Geometry check sheet. Reference: the model listing, model coordinates, mm. A direction names the side the tool comes from. Coordinates: 2 decimals unless noted, no trailing zeros. Write each loop counter-clockwise with the first axis right and the second up, starting at its lowest first coordinate (ties: lowest second). Pieces come first, ordered by that corner, then holes. Notation, with made-up numbers: (44, 54.25) -> (74, 54.25) arc R24 ccw to (74, 90.25) -> close; hole circle Ø11 at (33, 19.5). An arc over 180 degrees is marked (long way). Answer in a Markdown table with one row per item. Add a question column.
1. Cross-section at B-B on y = 5. Record the cut outline in (x, z) (3 decimals), and give its area (3 significant figures).
2. Cross-section at D-D on y = 28.5. Record the cut outline in (x, z) (3 decimals).
3. Cross-section at A-A on x = 0. Record the cut outline in (y, z) (3 decimals), and give its area (3 significant figures).
4. Mould release check, pull along X, two halves, no side actions. Record for faces 1 (the flat face through (0, 22.225, 136)), 2 (the flat face through (-1, 26, 0)), 3 (the flat face through (38.1, 38.1, 136.3)): pulls with the +X half, pulls with the -X half, needs draft (parallel to the pull), parting line crosses it, or undercut.
5. Cross-section at C-C on z = 114. Record the cut outline in (x, y) (3 decimals), and give its area (3 significant figures).
6. Depth check by flat-ended pin: P1, Ø8, axis at x = -28.575, z = 12.7, coming from the +Y side; P2, Ø7.5, axis at x = 3, z = 13.5, coming from the -Y side (3 decimals); P3, Ø24.5, axis at x = 32.5, z = 91, coming from the +Y side. Enter the tip coordinate at first touch or a pass-through.
7. Set-up check for faces 4 (the flat face through (41.275, 9, 74)), 5 (the cylindrical face through (30.318, 14.511, 121.915)), 6 (the flat face through (0, 22.225, 13)): record each of +Z, -Z, +X, -X, +Y, -Y from which the full face is reachable in a straight line by a thin tool's end or side.
8. Scan lines: L1, parallel to Z at x = 29, y = 7 (3 decimals); L2, parallel to Z at x = 28.5, y = 31 (3 decimals); L3, parallel to X at y = 5, z = 66 (3 decimals). Record each from-to range of solid material in increasing order. Write a range as from..to.
```python
from build123d import *

# Parameters (mm, degrees)
BOSS_EXTRUDE1_DEPTH     = 149.225
CHAMFER1_SIZE           = 6.35
F_3_8_CLEARANCE_HOLE1_D = 9.8044
SKETCH4_W               = 98.425
SKETCH4_H               = 28.575
CUT_EXTRUDE1_DEPTH      = 176.460048872
FILLET1_R               = 6.35
CUT_EXTRUDE2_START      = -123.825
SKETCH5_R               = 4.500000017
CUT_EXTRUDE2_DEPTH      = 40.64


with BuildPart() as part:
    # Sketch1 → Boss-Extrude1 (new body)
    with BuildSketch(Plane.XY):
        with BuildLine():
            Line((-19.05, 0), (-19.05, 19.05))
            ThreePointArc((-19.05, 19.05), (-18.12006403, 21.29506403), (-15.875, 22.225))
            Line((-15.875, 22.225), (15.875, 22.225))
            ThreePointArc((15.875, 22.225), (18.12006403, 21.29506403), (19.05, 19.05))
            Line((19.05, 19.05), (19.05, 0))
            Line((19.05, 0), (41.275, 0))
            Line((41.275, 0), (41.275, 41.275))
            Line((41.275, 41.275), (-41.275, 41.275))
            Line((-41.275, 41.275), (-41.275, 0))
            Line((-41.275, 0), (-19.05, 0))
        make_face()
    extrude(amount=BOSS_EXTRUDE1_DEPTH)

    # Chamfer1
    chamfer1_edges = [part.edges().sort_by_distance(p)[0] for p in [
        (-41.275, 41.275, 74.6125),
        (41.275, 41.275, 74.6125),
    ]]
    chamfer(chamfer1_edges, length=CHAMFER1_SIZE)

    # 3/8 Clearance Hole1 (through all)
    with Locations(Plane(origin=(0, 41.275, 0), x_dir=(1, 0, 0), z_dir=(0, 1, 0))):
        with Locations((28.575, -12.7), (-28.575, -136.525), (-28.575, -12.7), (28.575, -136.525)):
            Hole(F_3_8_CLEARANCE_HOLE1_D / 2)

    # Sketch4 → Cut-Extrude1 (cut, through all)
    with BuildSketch(Plane.ZY.offset(41.275)):
        with Locations((74.6125, 26.9875)):
            Rectangle(SKETCH4_W, SKETCH4_H)
    extrude(amount=-CUT_EXTRUDE1_DEPTH, mode=Mode.SUBTRACT)

    # Fillet1
    fillet1_edges = [part.edges().sort_by_distance(p)[0] for p in [
        (30.1625, 12.7, 25.4),
        (30.1625, 12.7, 123.825),
        (-30.1625, 12.7, 123.825),
        (-30.1625, 12.7, 25.4),
    ]]
    fillet(fillet1_edges, radius=FILLET1_R)

    # Sketch5 → Cut-Extrude2 (cut)
    with BuildSketch(Plane.XY.offset(149.225).offset(CUT_EXTRUDE2_START)):
        with Locations((0, 31.115)):
            Circle(SKETCH5_R)
    extrude(amount=-CUT_EXTRUDE2_DEPTH, mode=Mode.SUBTRACT)


solid = part.part
```
Results found:
| question | item | result |
|---|---|---|
| 1 | outline | (-41.275, 0) -> (-19.05, 0) -> (-19.05, 149.225) -> (-41.275, 149.225) -> close; (19.05, 0) -> (41.275, 0) -> (41.275, 149.225) -> (19.05, 149.225) -> close; hole circle Ø9.804 at (-28.575, 12.7); hole circle Ø9.804 at (-28.575, 136.525); hole circle Ø9.804 at (28.575, 12.7); hole circle Ø9.804 at (28.575, 136.525) |
| 1 | area | 6,330 mm^2 |
| 2 | outline | (-41.275, 0) -> (-3.662, 0) -> (-3.662, 25.4) -> (-41.275, 25.4) -> close; (-41.275, 123.825) -> (41.275, 123.825) -> (41.275, 149.225) -> (-41.275, 149.225) -> close; (3.662, 0) -> (41.275, 0) -> (41.275, 25.4) -> (3.662, 25.4) -> close; hole circle Ø9.804 at (-28.575, 12.7); hole circle Ø9.804 at (-28.575, 136.525); hole circle Ø9.804 at (28.575, 12.7); hole circle Ø9.804 at (28.575, 136.525) |
| 3 | outline | (22.225, 0) -> (26.615, 0) -> (26.615, 25.4) -> (22.225, 25.4) -> close; (22.225, 123.825) -> (41.275, 123.825) -> (41.275, 149.225) -> (22.225, 149.225) -> close; (35.615, 0) -> (41.275, 0) -> (41.275, 25.4) -> (35.615, 25.4) -> close |
| 3 | area | 739 mm^2 |
| 4 | face 1 | undercut |
| 4 | face 2 | needs draft |
| 4 | face 3 | pulls with the +X half |
| 5 | outline | (-41.275, 0) -> (-19.05, 0) -> (-19.05, 12.7) -> (-41.275, 12.7) -> close; (19.05, 0) -> (41.275, 0) -> (41.275, 12.7) -> (19.05, 12.7) -> close |
| 5 | area | 565 mm^2 |
| 6 | P1 | passes through |
| 6 | P2 | stops at y = 22.225 |
| 6 | P3 | stops at y = 12.7 |
| 7 | face 4 | +Z, -Z, +X, +Y, -Y |
| 7 | face 5 | +X, -X, +Y |
| 7 | face 6 | +Z, -Z, -Y |
| 8 | L1 | z = 0..7.816, 17.584..131.641, 141.409..149.225 |
| 8 | L2 | z = 0..7.798, 17.602..25.4, 123.825..131.623, 141.427..149.225 |
| 8 | L3 | x = -41.275..-19.05, 19.05..41.275 |
